Geometry: final body of the model. Coordinates: model frame, mm. A direction names the side the tool comes from. Coordinates: 2 decimals unless noted, no trailing zeros. Order: outer loops, then holes, each group sorted by start corner. A loop starts at its lowest first (then second) coordinate and runs counter-clockwise, first axis right, second up. Notation, with made-up numbers: (-12, 69) -> (0, 69) arc R26 cw to (0, 98) -> close; hole circle Ø2 at (70.5, 61). An arc over 180 degrees is marked (long way). Answer in a Markdown table with one row per item. Add a question column.
1) Contact query for flat-ended pins moving along their axis: P1, Ø2, axis at y = -46.5, z = -5.5, coming from the -X side; P2, Ø8, axis at x = 5.5, z = -1, coming from the -Y side; P3, Ø5, axis at y = 14.5, z = -18.5, coming from the -X side. Output: stop coordinate, or through.
2) Ray query, line 1 (Y direction, x = 0, z = -19); line 2 (Y direction, x = 0, z = 7.75); line 3 (Z direction, x = 60, y = 59). Return the intervals inside material, ascending. Write a range as from..to.
3) Pull-direction query (Y, two-part tool) for faces 1 (the face through (-52, 81, 38.1)), 2 (the face through (-22.025, -99.184, 0.498)), 3 (the face through (-1, -40, 12.7)); classes: +Y half, -Y half, draft (parallel to the pull), parting line (faces both ways), or undercut.
4) Section query A-A on y = 0. Return the cut outline in (x, z), then the cut area to 3 significant figures.
5) Set-up query: faces 4 (the face through (-52, 81, -38.1)), 5 (the face through (-12.096, 92.128, 24.29)), 6 (the face through (-12.096, 92.128, -24.29)). Return all of +Z, -Z, +X, -X, +Y, -Y with unobstructed straight access to the full face (end or side cutting, diameter ignored); none if empty.
6) Section query C-C on z = -31.5. Return the cut outline in (x, y), then the cut area to 3 significant figures.
```python
from build123d import *

# Parameters (mm, degrees)
SKETCH1_R           = 101.6
SKETCH1_R_2         = 31.75
BOSS_EXTRUDE1_DEPTH = 38.1
SKETCH2_R           = 92.918511566
CUT_EXTRUDE1_DEPTH  = 25.4
FILLET1_R           = 2.54
FILLET2_R           = 2.54


with BuildPart() as part:
    # Sketch1 → Boss-Extrude1 (new, symmetric)
    with BuildSketch(Plane.XY):
        Circle(SKETCH1_R)
        Circle(SKETCH1_R_2, mode=Mode.SUBTRACT)
    extrude(amount=BOSS_EXTRUDE1_DEPTH, both=True)

    # Sketch2 → Cut-Extrude1 (cut)
    with BuildSketch(Plane.XY.offset(38.1)):
        Circle(SKETCH2_R)
    cut_extrude1 = extrude(amount=-CUT_EXTRUDE1_DEPTH, mode=Mode.SUBTRACT)

    # Mirror1: Cut-Extrude1 across plane
    add(cut_extrude1.mirror(Plane.XY), mode=Mode.SUBTRACT)

    # Fillet1
    fillet1_edges = [part.edges().sort_by_distance(p)[0] for p in [
        (-92.918511566, 0, -38.1),
        (-101.6, 0, -38.1),
    ]]
    fillet(fillet1_edges, radius=FILLET1_R)

    # Fillet2
    fillet2_edges = [part.edges().sort_by_distance(p)[0] for p in [
        (-92.918511566, 0, 38.1),
        (-101.6, 0, 38.1),
    ]]
    fillet(fillet2_edges, radius=FILLET2_R)


solid = part.part
```
Result:
| question | item | result |
|---|---|---|
| 1 | P1 | x = -90.84 |
| 1 | P2 | y = -101.59 |
| 1 | P3 | x = -100.89 |
| 2 | line 1 | -101.6..-92.92, 92.92..101.6 |
| 2 | line 2 | -101.6..-31.75, 31.75..101.6 |
| 2 | line 3 | -12.7..12.7 |
| 3 | face 1 | draft |
| 3 | face 2 | parting line |
| 3 | face 3 | undercut |
| 4 | outline | (-101.6, -35.56) arc R2.54 ccw to (-99.06, -38.1) -> (-95.46, -38.1) arc R2.54 ccw to (-92.92, -35.56) -> (-92.92, -12.7) -> (-31.75, -12.7) -> (-31.75, 12.7) -> (-92.92, 12.7) -> (-92.92, 35.56) arc R2.54 ccw to (-95.46, 38.1) -> (-99.06, 38.1) arc R2.54 ccw to (-101.6, 35.56) -> close; (31.75, -12.7) -> (92.92, -12.7) -> (92.92, -35.56) arc R2.54 ccw to (95.46, -38.1) -> (99.06, -38.1) arc R2.54 ccw to (101.6, -35.56) -> (101.6, 35.56) arc R2.54 ccw to (99.06, 38.1) -> (95.46, 38.1) arc R2.54 ccw to (92.92, 35.56) -> (92.92, 12.7) -> (31.75, 12.7) -> close |
| 4 | area | 4,420 mm2 |
| 5 | face 4 | -Z, +X, -X, +Y, -Y |
| 5 | face 5 | +Z |
| 5 | face 6 | -Z |
| 6 | outline | circle Ø203.2 at (0, 0); hole circle Ø185.84 at (0, 0) |
| 6 | area | 5,310 mm2 |
